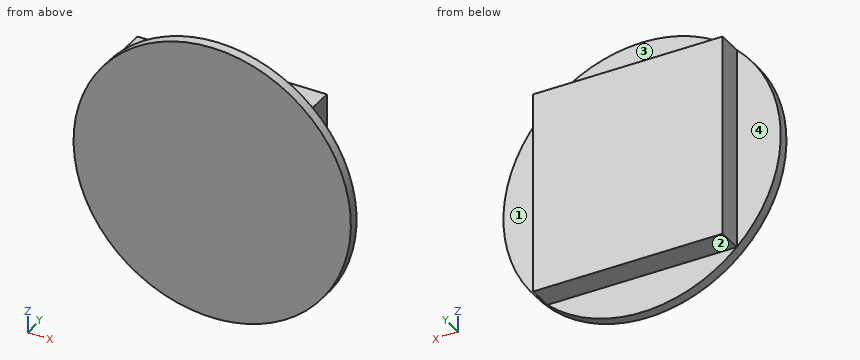
```python
from build123d import *

# Parameters (mm, degrees)
BOSS_EXTRUDE1_DEPTH      = 10
BOSS_EXTRUDE1_DEPTH_BACK = 10
SKETCH1_R                = 277.5
SKETCH2_W                = 378.949229626
SKETCH2_H                = 405.490420806
BOSS_EXTRUDE2_DEPTH      = 50


with BuildPart() as part:
    # Sketch1 → Boss-Extrude1 (new, two sides: drawn at the far end of the back side and taken through both)
    with BuildSketch(Plane(origin=(0, 0, 0), x_dir=(1, 0, 0), z_dir=(0, 1, 0)).offset(-BOSS_EXTRUDE1_DEPTH_BACK)):
        with Locations(Location((0, 0, 0), (0, 0, 270))):
            Circle(SKETCH1_R)
    extrude(amount=BOSS_EXTRUDE1_DEPTH + BOSS_EXTRUDE1_DEPTH_BACK)

    # Sketch2 → Boss-Extrude2 (add)
    with BuildSketch(Plane(origin=(0, 10, 0), x_dir=(1, 0, 0), z_dir=(0, 1, 0))):
        Rectangle(SKETCH2_W, SKETCH2_H)
    extrude(amount=BOSS_EXTRUDE2_DEPTH)


solid = part.part
```
Verification items for the finished model (mm, model axes). Face numbers are marked on the shaded views. A direction names the side the tool comes from. Coordinates: 2 decimals unless noted, no trailing zeros. Loops run counter-clockwise (first coordinate to the right, second up) from the corner with the lowest first, then second, coordinate; pieces in that order, holes last. Notation, with made-up numbers: (60.5, 6.25) - (96.5, 6.25) arc R23 ccw to (96.5, 31.25) - close; hole circle Ø6 at (82, 24.5). An arc over 180 degrees is marked (long way). Return JSON: item names as keys, results as strings.
1. Section check D-D, the plane y = 1. Record the boundary of the cut face in (x, z).
Established:
{"outline": "circle Ø555 at (0, 0)"}
2. Go/stop test with flat-tipped pins: pin 1 (1 mm diameter, centred on y = -0.5, z = 96.5, fed in from +X); pin 2 (25 mm diameter, centred on x = 22.5, y = 27, fed in from +Z); pin 3 (6 mm diameter, centred on x = 137, y = 50, fed in from -Z). Record where each tip stops, or that it passes through.
Established:
{"pin 1": "stops at x = 260.37", "pin 2": "stops at z = 202.75", "pin 3": "stops at z = -202.75"}
3. Section check B-B, the plane z = 0. Record the boundary of the cut face in (x, y).
Established:
{"outline": "(-277.5, -10) - (277.5, -10) - (277.5, 10) - (189.47, 10) - (189.47, 60) - (-189.47, 60) - (-189.47, 10) - (-277.5, 10) - close"}
4. Section check C-C, the plane y = 52. Record the boundary of the cut face in (x, z), then the cut area to 3 significant figures.
Established:
{"outline": "(-189.47, -202.75) - (189.47, -202.75) - (189.47, 202.75) - (-189.47, 202.75) - close", "area": "154,000 mm2"}
5. Tool access check on the marked faces 1, 2, 3 and 4. Record the directions out of +Z, -Z, +X, -X, +Y, -Y that give a thin tool (end or side, any length) a straight path to the whole face; none if there is none.
Established:
{"face 1": "+Z, -Z, +X, +Y", "face 2": "-Z, +X, -X, +Y", "face 3": "+Z, +X, -X, +Y", "face 4": "+Z, -Z, -X, +Y"}
6. Section check A-A, the plane x = 0. Record the boundary of the cut face in (y, z).
Established:
{"outline": "(-10, -277.5) - (10, -277.5) - (10, -202.75) - (60, -202.75) - (60, 202.75) - (10, 202.75) - (10, 277.5) - (-10, 277.5) - close"}
7. Thickness scan on L1, parallel to Z at x = -143.5, y = 41; L2, parallel to X at y = 50.5, z = 189.5; L3, parallel to Y at x = 223.5, z = 9. Record the ranges inside material, lowest first.
Established:
{"L1": "z = -202.75 to 202.75", "L2": "x = -189.47 to 189.47", "L3": "y = -10 to 10"}
